Can you work these out from the model? Positions are in its coordinate system, mm. A direction names the side the tool comes from. Give positions to 0.01 mm unless a question says otherwise; leave off trailing zeros. Loops run counter-clockwise (first coordinate to the right, second up) from the corner with the lowest first, then second, coordinate; pieces in that order, holes last. Notation, with made-up numbers: (-5.5, 50) -> (41.5, 50) arc R16 ccw to (41.5, 75) -> close; hole circle Ø6 at (-11, 49). An arc over 180 degrees is marked (long way). One line per question, with ' | ' between items.
Autodesk Inventor part; units mm, degrees
ref_plane "YZ Plane" through (0, 0, 0) normal (1, 0, 0) x (0, 1, 0)
ref_plane "XZ Plane" through (0, 0, 0) normal (0, 1, 0) x (-1, 0, 0)
ref_plane "XY Plane" through (0, 0, 0) normal (0, 0, 1) x (1, 0, 0)
sketch "Sketch1" plane through (0, 0, 0) normal (0, 1, 0) x (-1, 0, 0)
  line L0 (16.5, 4) -> (12.5, 4)
  line L1 (12.5, 4) -> (12.5, -4)
  line L2 (12.5, -4) -> (16.5, -4)
  line L3 (16.5, -2.5) -> (40, -2.5)
  line L4 (40, 2.5) -> (16.5, 2.5)
  line L5 (40, 4) -> (45, 4)
  line L6 (45, 4) -> (45, -4)
  line L7 (45, -4) -> (40, -4)
  line L8 (16.5, 2.5) -> (16.5, 4)
  line L9 (16.5, -4) -> (16.5, -2.5)
  line L10 (40, -4) -> (40, -2.5)
  line L11 (40, 2.5) -> (40, 4)
  line L12 (0, -5.6) -> (0, 5.6)
  line L13 (45, 4) -> (12.5, -4) construction
  line L14 (45, -4) -> (12.5, 4) construction
  point P0 (0, 0)
  point P1 (45, 0)
  point P2 (28.75, 0)
  point P3 (40, 2)
  point P4 (16.5, -2)
  point P5 (40, -2)
  point P6 (16.5, 2)
  dimension "d1" = 90
  dimension "d2" = 5
  dimension "d3" = 4
  dimension "d4" = 25
  dimension "d5" = 8
  dimension "d7" = 1.5
revolve "Revolution1" add sketch "Sketch1" angle 360 about axis through (0, 0, -10) along (0, 0, 1)
properties part number "Counterweight (500g)" material "Steel, Cast"
Q1. For pin 1 Ø12 at (x, y) = (22.5, 17) entering from +Z; pin 2 Ø1 at (x, z) = (-1.5, -1) entering from -Y; pin 3 Ø8 at (x, y) = (-11.5, 19) entering from -Z, each with a flat end and sliding along its axis, tell me the tip position at first contact or that it passes through.
Entries:
pin 1: z = 2.5 | pin 2: y = -44.99 | pin 3: z = -2.5
Q2. If we section it at D-D (y = -20): Write out the boundary of the cut face in (x, z).
Entries:
outline: (-40.31, -4) -> (-34.64, -4) -> (-34.64, -2.5) -> (34.64, -2.5) -> (34.64, -4) -> (40.31, -4) -> (40.31, 4) -> (34.64, 4) -> (34.64, 2.5) -> (-34.64, 2.5) -> (-34.64, 4) -> (-40.31, 4) -> close
Q3. If we mould it in two halves opening along Y, with no side actions, what happens to faces 1 (the face through (-20.765, -39.923, -0.056)), 2 (the face through (-17, -1, 2.5)), 3 (the face through (12.3, -3.7, 4))? For each: pulls with the +Y half, pulls with the -Y half, needs draft (parallel to the pull), parting line crosses it, or undercut.
Entries:
face 1: parting line crosses it | face 2: undercut | face 3: needs draft
Q4. If we section it at C-C (x = 22): Write out the boundary of the cut face in (y, z).
Entries:
outline: (-39.26, -4) -> (-33.41, -4) -> (-33.41, -2.5) -> (33.41, -2.5) -> (33.41, -4) -> (39.26, -4) -> (39.26, 4) -> (33.41, 4) -> (33.41, 2.5) -> (-33.41, 2.5) -> (-33.41, 4) -> (-39.26, 4) -> close
Q5. If we section it at A-A (x = 0): Write out the boundary of the cut face in (y, z).
Entries:
outline: (-45, -4) -> (-40, -4) -> (-40, -2.5) -> (-16.5, -2.5) -> (-16.5, -4) -> (-12.5, -4) -> (-12.5, 4) -> (-16.5, 4) -> (-16.5, 2.5) -> (-40, 2.5) -> (-40, 4) -> (-45, 4) -> close; (12.5, -4) -> (16.5, -4) -> (16.5, -2.5) -> (40, -2.5) -> (40, -4) -> (45, -4) -> (45, 4) -> (40, 4) -> (40, 2.5) -> (16.5, 2.5) -> (16.5, 4) -> (12.5, 4) -> close
Q6. If I drill on probe 1 along X at (y, z) = (0, 3.5); probe 2 along Y at (x, z) = (0, 1.5), over which ranges is the centre line in solid material (lowest first)? Write a range as from..to.
Entries:
probe 1: -45..-40, -16.5..-12.5, 12.5..16.5, 40..45 | probe 2: -45..-12.5, 12.5..45
Q7. On a 3-axis mill with a long thin cutter (end or side, diameter ignored), from which of +Z, -Z, +X, -X, +Y, -Y can I reach the whole of each face in a straight line? I mean faces 4 (the face through (-11.923, 3.755, -0.056)), 5 (the face through (8.67, 39.05, 3.26)), 6 (the face through (-17, -1, -2.5)). Say none if no direction works.
Entries:
face 4: +Z, -Z | face 5: +Z | face 6: -Z
